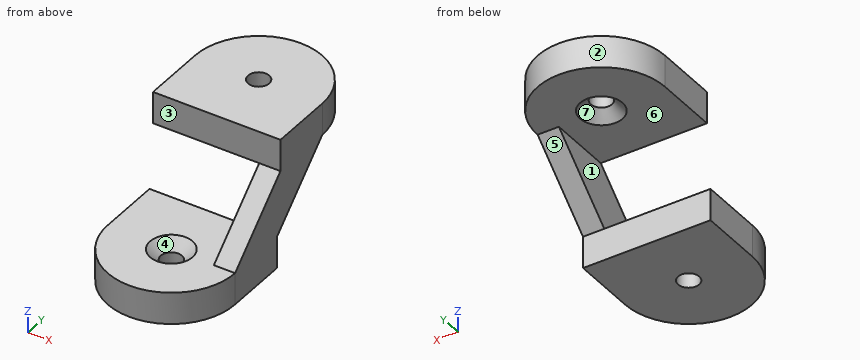
```python
from build123d import *

# Parameters (mm, degrees)
SKETCH_R     = 2
PAD_DEPTH    = 6
PAD001_DEPTH = 4
SKETCH004_R  = 2
PAD002_DEPTH = 6
CHAMFER_SIZE = 2


with BuildPart() as part:
    # Sketch → Pad (new body)
    with BuildSketch(Plane.XY):
        with BuildLine():
            Line((-12, 0), (-12, 12))
            Line((-12, 12), (12, 12))
            Line((12, 12), (12, 0))
            ThreePointArc((-12, 0), (0, -12), (12, 0))
        make_face()
        Circle(SKETCH_R, mode=Mode.SUBTRACT)
    extrude(amount=PAD_DEPTH)

    # Sketch003 (on Face3 of Pad) → Pad001 (join)
    with BuildSketch(Plane.YZ.offset(12)):
        Polygon((0, 6), (13, 18), (25, 18), (12, 6), align=None)
    extrude(amount=-PAD001_DEPTH)

    # Sketch004 (on Face12 of Pad001) → Pad002 (join)
    with BuildSketch(Plane.XY.offset(18)):
        with BuildLine():
            Line((12, 25), (12, 13))
            Line((12, 13), (-12, 13))
            Line((-12, 13), (-12, 25))
            ThreePointArc((12, 25), (0, 37), (-12, 25))
        make_face()
        with Locations((0, 25)):
            Circle(SKETCH004_R, mode=Mode.SUBTRACT)
    extrude(amount=PAD002_DEPTH)

    # Chamfer
    chamfer_edges = [part.edges().sort_by_distance(p)[0] for p in [
        (-2, 0, 6),
        (-2, 25, 18),
    ]]
    chamfer(chamfer_edges, length=CHAMFER_SIZE)


solid = part.part
```
Work out the finished part from the listing and answer in its coordinate system (mm). Face numbers are marked on the shaded views. A direction names the side the tool comes from. Give positions to 0.01 mm unless a question says otherwise; leave off trailing zeros. Loops run counter-clockwise (first coordinate to the right, second up) from the corner with the lowest first, then second, coordinate; pieces in that order, holes last. Notation, with made-up numbers: (65.5, -33) -> (109.5, -33) arc R12 cw to (109.5, -11) -> close; hole circle Ø1 at (84, 72.25). An arc over 180 degrees is marked (long way). Use CSV: the item, a comma, the result in double quotes.
1. The part is cut by section B-B (x = 9.75). Write down the section's boundary in (y, z).
Found:
outline,"(-7, 0) -> (12, 0) -> (12, 6) -> (25, 18) -> (32, 18) -> (32, 24) -> (13, 24) -> (13, 18) -> (0, 6) -> (-7, 6) -> close"
2. The part is cut by section A-A (x = 0). Write down the section's boundary in (y, z).
Found:
outline,"(-12, 0) -> (-2, 0) -> (-2, 4) -> (-4, 6) -> (-12, 6) -> close; (2, 0) -> (12, 0) -> (12, 6) -> (4, 6) -> (2, 4) -> close; (13, 18) -> (21, 18) -> (23, 20) -> (23, 24) -> (13, 24) -> close; (27, 20) -> (29, 18) -> (37, 18) -> (37, 24) -> (27, 24) -> close"
3. The part is cut by section C-C (y = 7). Write down the section's boundary in (x, z), then the cut area to 3 significant figures.
Found:
outline,"(-12, 0) -> (12, 0) -> (12, 12.46) -> (8, 12.46) -> (8, 6) -> (-12, 6) -> close"
area,"170 mm^2"
4. A tool of negligible diameter and unlimited length cuts with its end or side. For the marked faces 1, 2 and 3, from which of +Z, -Z, +X, -X, +Y, -Y can it reach the whole face along a straight path? Write none if from no direction.
Found:
face 1,"-X, +Y, -Y"
face 2,"+Z, -Z, +Y"
face 3,"+Z, +X, -X, -Y"
5. Flat-ended cylindrical pins translate along their axes: pin 1 Ø3 at (x, y) = (-1.5, 19.5) entering from -Z; pin 2 Ø6.5 at (x, z) = (4.5, 19.5) entering from -Y; pin 3 Ø7 at (x, y) = (4, 6) entering from +Z. Find the tip coordinate at first contact, or state that the pin passes through.
Found:
pin 1,"z = 18"
pin 2,"y = 13"
pin 3,"z = 6"
6. The part is cut by section D-D (z = 10.5). Write down the section's boundary in (x, y) (3 decimals), then the cut area to 3 significant figures.
Found:
outline,"(8, 4.875) -> (12, 4.875) -> (12, 16.875) -> (8, 16.875) -> close"
area,"48.0 mm^2"
7. Straight lines are drawn through the part: line 1 (Y direction, x = 0, z = 1.85); line 2 (Y direction, x = 0, z = 22.5); line 3 (X direction, y = 10, z = 7.25). For each, find the intervals that lie inside material, in ascending order.
Found:
line 1,"-12 to -2, 2 to 12"
line 2,"13 to 23, 27 to 37"
line 3,"8 to 12"
8. The mould has two halves that part along Y. Classify the marked faces 4, 5, 6 and 7: +Y half, -Y half, draft (parallel to the pull), parting line (faces both ways), or undercut.
Found:
face 4,"undercut"
face 5,"+Y half"
face 6,"draft"
face 7,"undercut"
